Here's how the part is built. I have some questions about the finished solid (model axes, mm). A direction names the side the tool comes from. Round coordinates to 2 decimals unless told otherwise and drop trailing zeros. Loops run counter-clockwise (first coordinate to the right, second up) from the corner with the lowest first, then second, coordinate; pieces in that order, holes last. Notation, with made-up numbers: (64.5, 60) - (120.5, 60) arc R20 cw to (120.5, 69) - close; hole circle Ø4 at (-30.75, 21.25). An arc over 180 degrees is marked (long way). Return JSON: item names as keys, results as strings. Group by question number.
Autodesk Inventor part; units mm, degrees
ref_plane "Work Plane1" through (0, 110.0074, 0) normal (0, 1, 0) x (-1, 0, 0)
ref_plane "YZ Plane" through (0, 0, 0) normal (1, 0, 0) x (0, 1, 0)
ref_plane "XY Plane" through (0, 0, 0) normal (0, 0, 1) x (1, 0, 0)
sketch "Sketch1" plane through (0, 0, 0) normal (0, 1, 0) x (-1, 0, 0)
  line L0 (49.5033, -49.5033) -> (-60.5041, -49.5033)
  line L1 (-60.5041, -49.5033) -> (-60.5041, 60.5041)
  line L2 (-60.5041, 60.5041) -> (49.5033, 60.5041)
  line L3 (49.5033, 60.5041) -> (49.5033, -49.5033)
  point P0 (0, 0)
  dimension "d0" = 110.0074
extrude "Extrusion1" add sketch "Sketch1" along normal blind 110.0074
ref_plane "Work Plane1" through (0, 110.0074, 0) normal (0, 1, 0) x (-1, 0, 0)
sketch "Sketch2" plane through (0, 110.0074, 0) normal (0, 1, 0) x (-1, 0, 0)
  circle A0 centre (-5.5004, 5.5977) radius 9.4996
  line L0 (-60.5041, 60.5041) -> (-60.5041, -49.5033)
  line L1 (49.5033, -49.5033) -> (49.5033, 60.5041)
  line L2 (-2.3762, -7.0261) -> (-8.6246, -7.0261)
  line L3 (-8.6246, -7.0261) -> (-8.6246, -3.3735)
  line L4 (-2.3762, -7.0261) -> (-2.3762, -3.3735)
  point P0 (0, 0)
  dimension "d4" = 18.9992
  dimension "d5" = 55.0037
  dimension "d8" = 6.2484
  dimension "d9" = 3.1242
extrude "Extrusion2" add sketch "Sketch2" along normal blind 56.007
properties part number "MainMotor"
Q1. For faces 1 (the cylindrical face through (5.87, 137.62, 15.09)), 2 (the flat face through (5, 138, -7.026)), 3 (the flat face through (6, 54, 60.504)), 4 (the flat face through (8.625, 138, -5)), 5 (the flat face through (2.376, 138, -5)), which set-ups out of +Z, -Z, +X, -X, +Y, -Y let a thin tool reach every point of the face, with its end or its side?
Q2. Please list where these lines run through material, in increasing order: line 1 (Y direction, x = 51.5, z = 34); line 2 (Z direction, x = 14, y = 124.5).
Q3. Will these pins go through, and if not, where does the flat tip stop? pin 1 Ø1.9 at (x, y) = (4.5, 144.5) entering from -Z; pin 2 Ø1.8 at (y, z) = (150, -4.5) entering from -X; pin 3 Ø4 at (x, z) = (14.5, -6.5) entering from -Y; pin 4 Ø4 at (y, z) = (140.5, -5) entering from +X.
Q4. Imagine slicing it at B-B, the plane z = -30.5. List the corners of the cut face in (x, y) for me, and give its area (3 significant figures).
Q5. Imagine slicing it at A-A, the plane x = 11.5. List the corners of the cut face in (y, z) for me, and give its area (3 significant figures).
Q6. Imagine slicing it at C-C, the plane y = 153.5. List the corners of the cut face in (x, z) for me.
Output values:
{
 "1": {"face 1": "+Y", "face 2": "-Z, +X, -X, +Y", "face 3": "+Z, +X, -X, +Y, -Y", "face 4": "-Z, +X, +Y", "face 5": "-Z, -X, +Y"},
 "2": {"line 1": "y = 0 to 110.01", "line 2": "z = 1.36 to 9.84"},
 "3": {"pin 1": "stops at z = -7.03", "pin 2": "stops at x = 2.38", "pin 3": "stops at y = 0", "pin 4": "stops at x = 9.54"},
 "4": {"outline": "(-49.5, 0) - (60.5, 0) - (60.5, 110.01) - (-49.5, 110.01) - close", "area": "12,100 mm^2"},
 "5": {"outline": "(0, -49.5) - (110.01, -49.5) - (110.01, -1.77) - (166.01, -1.77) - (166.01, 12.96) - (110.01, 12.96) - (110.01, 60.5) - (0, 60.5) - close", "area": "12,900 mm^2"},
 "6": {"outline": "(2.38, -7.03) - (8.62, -7.03) - (8.62, -3.37) arc R9.5 ccw (long way) to (2.38, -3.37) - close"}
}
